Here's how the part is built. I have some questions about the finished solid (model axes, mm). A direction names the side the tool comes from. Coordinates: 2 decimals unless noted, no trailing zeros. Write each loop counter-clockwise with the first axis right and the second up, starting at its lowest first coordinate (ties: lowest second). Pieces come first, ordered by that corner, then holes. Notation, with made-up numbers: (33.25, 17.5) - (84.25, 17.5) arc R20 ccw to (84.25, 46.5) - close; hole circle Ø6 at (70, -27). An arc over 180 degrees is marked (long way). Answer in a Markdown table with one row per item. Add a question column.
Item 1: Imagine slicing it at B-B (y = 11). Please give me the cut outline in (x, z), plus the area to 3 significant figures.
Item 2: We'd pull the mould along Z, two halves only. Please class faces 1 (the face through (-1, 10, -38.1)), 2 (the face through (-1, 0, -1)), 3 (the face through (0, 17.78, 0)): +Z half, -Z half, draft (parallel to the pull), parting line (faces both ways), or undercut.
Item 3: If I drill on probe 1 along Z at (x, y) = (16, 11); probe 2 along Y at (x, z) = (7, -27), over which ranges is the centre line in solid material (lowest first)? Write a range as from..to.
Item 4: I'm going to push a flat-ended pin straight in: pin 1 (8 mm diameter, centred on x = 9, z = 18.5, fed in from -Y). Where does the tip first touch, or does it pass through?
Item 5: Which directions (+Z, -Z, +X, -X, +Y, -Y) give clear straight access to the entire face, cutting with the end or side of a thin tool? Please do faces 4 (the face through (-1, 10, 38.1)), 5 (the face through (0, 10, -35.56)).
Item 6: Imagine slicing it at A-A (x = 25). Please give me the cut outline in (y, z).
from build123d import *

# Parameters (mm, degrees)
SKETCH1_W           = 76.2
SKETCH1_H           = 76.2
BOSS_EXTRUDE3_DEPTH = 20.32
SHELL3_T            = 2.54


with BuildPart() as part:
    # Sketch1 → Boss-Extrude3 (new body)
    with BuildSketch(Plane(origin=(0, 0, 0), x_dir=(1, 0, 0), z_dir=(0, 1, 0))):
        Rectangle(SKETCH1_W, SKETCH1_H)
    extrude(amount=BOSS_EXTRUDE3_DEPTH)

    # Shell3 (no face opened: a closed hollow body)
    add(offset(amount=-SHELL3_T, mode=Mode.PRIVATE), mode=Mode.SUBTRACT)


solid = part.part
Here are the results:
| question | item | result |
|---|---|---|
| 1 | outline | (-38.1, -38.1) - (38.1, -38.1) - (38.1, 38.1) - (-38.1, 38.1) - close; hole (-35.56, -35.56) - (35.56, -35.56) - (35.56, 35.56) - (-35.56, 35.56) - close |
| 1 | area | 748 mm2 |
| 2 | face 1 | -Z half |
| 2 | face 2 | draft |
| 2 | face 3 | undercut |
| 3 | probe 1 | z = -38.1..-35.56, 35.56..38.1 |
| 3 | probe 2 | y = 0..2.54, 17.78..20.32 |
| 4 | pin 1 | stops at y = 0 |
| 5 | face 4 | +Z, +X, -X, +Y, -Y |
| 5 | face 5 | none |
| 6 | outline | (0, -38.1) - (20.32, -38.1) - (20.32, 38.1) - (0, 38.1) - close; hole (2.54, -35.56) - (17.78, -35.56) - (17.78, 35.56) - (2.54, 35.56) - close |
